from build123d import *

# Parameters (mm, degrees)
SKETCH1_R           = 4
SKETCH1_R_2         = 1
BOSS_EXTRUDE1_DEPTH = 1
FILLET1_R           = 2


with BuildPart() as part:
    # Sketch1 → Boss-Extrude1 (new body)
    with BuildSketch(Plane.XY):
        Polygon((-31.163774815, -36.354373739), (-22.29015667, -20.984816263), (-9.5, -16.574119451), (-9.5, 20), (9.5, 20), (9.5, -18.535898385), (1.11843014, -33.05320323), (12.977241336, -39.899891067), (3.477241336, -56.354373739), align=None)
        with Locations((0, 10.5)):
            Circle(SKETCH1_R, mode=Mode.SUBTRACT)
        with Locations((0, -43.377132403)):
            Circle(SKETCH1_R, mode=Mode.SUBTRACT)
        with Locations((2.745190528, -53.622322931)):
            Circle(SKETCH1_R_2, mode=Mode.SUBTRACT)
        with Locations((-28.431724008, -35.622322931)):
            Circle(SKETCH1_R_2, mode=Mode.SUBTRACT)
        with Locations((10.245190528, -40.631941874)):
            Circle(SKETCH1_R_2, mode=Mode.SUBTRACT)
        with Locations((-20.931724008, -22.631941874)):
            Circle(SKETCH1_R_2, mode=Mode.SUBTRACT)
        with Locations((-7.5, -18)):
            Circle(SKETCH1_R_2, mode=Mode.SUBTRACT)
        with Locations((7.5, -18)):
            Circle(SKETCH1_R_2, mode=Mode.SUBTRACT)
        with Locations((7.5, 18)):
            Circle(SKETCH1_R_2, mode=Mode.SUBTRACT)
        with Locations((-7.5, 18)):
            Circle(SKETCH1_R_2, mode=Mode.SUBTRACT)
    extrude(amount=BOSS_EXTRUDE1_DEPTH)

    # Fillet1
    fillet1_edges = [part.edges().sort_by_distance(p)[0] for p in [
        (-22.29015667, -20.984816263, 0.5),
        (-9.5, -16.574119451, 0.5),
        (-9.5, 20, 0.5),
        (9.5, 20, 0.5),
        (9.5, -18.535898385, 0.5),
        (1.11843014, -33.05320323, 0.5),
        (12.977241336, -39.899891067, 0.5),
        (3.477241336, -56.354373739, 0.5),
        (-31.163774815, -36.354373739, 0.5),
    ]]
    fillet(fillet1_edges, radius=FILLET1_R)


solid = part.part
Geometry check sheet. Reference: the model listing, model coordinates, mm. A direction names the side the tool comes from. Give positions to 0.01 mm unless a question says otherwise; leave off trailing zeros. Loops run counter-clockwise (first coordinate to the right, second up) from the corner with the lowest first, then second, coordinate; pieces in that order, holes last. Notation, with made-up numbers: M -24.75,28.5 L -15.75,28.5 A15 ccw -15.75,56.5 Z; hole C -38.75,-11.5 d9. An arc over 180 degrees is marked long. Answer as a JSON object with one key per item and string values. Group by question number.
Item 1: Mould release check, pull along Y, two halves, no side actions. Record for faces 3 (the cylindrical face through (8.9, 19.43, 0.51)), 4 (the cylindrical face through (2.53, -54.6, 0.49)), 5 (the flat face through (8.3, -48, 0.5)), 6 (the cylindrical face through (9.246, -40.588, 0.493)): pulls with the +Y half, pulls with the -Y half, needs draft (parallel to the pull), parting line crosses it, or undercut.
Item 2: Material ranges on L1, parallel to Y at x = 0, z = 0.3; L2, parallel to Y at x = 7.5, z = 0.75; L3, parallel to Y at x = -1, z = 0.75, recorded low to high.
Item 3: Sectioned sample at D-D on x = -18. Record the boundary of the cut face in (y, z).
Item 4: Sectioned sample at A-A on y = 11.5. Record the boundary of the cut face in (x, z), plus the area to 3 significant figures.
Item 5: Access from +Z, -Z, +X, -X, +Y, -Y to the whole of each face (thin tool, end or side, straight path). Record for faces 1 (the cylindrical face through (-7.717, -18.976, 0.493)), 2 (the flat face through (6.989, -36.443, 0.493)).
Item 6: Sectioned sample at C-C on z = 0.75. Give the number of separate pieces and of enclosed holes in the cut face, plus the area to 3 significant figures.
Item 7: Sectioned sample at B-B on x = 0. Record the boundary of the cut face in (y, z).
Findings below:
{
 "1": {"face 3": "pulls with the +Y half", "face 4": "undercut", "face 5": "pulls with the -Y half", "face 6": "undercut"},
 "2": {"L1": "-54.35 to -47.38, -39.38 to 6.5, 14.5 to 20", "L2": "-49.39 to -36.74, -22 to -19, -17 to 17, 19 to 20", "L3": "-53.77 to -47.25, -39.5 to 6.63, 14.37 to 20"},
 "3": {"outline": "M -43.95,0 L -19.51,0 L -19.51,1 L -43.95,1 Z"},
 "4": {"outline": "M -9.5,0 L -3.87,0 L -3.87,1 L -9.5,1 Z; M 3.87,0 L 9.5,0 L 9.5,1 L 3.87,1 Z", "area": "11.3 mm2"},
 "5": {"face 1": "+Z, -Z", "face 2": "+Z, -Z, +X"},
 "6": {"separate pieces": "1", "enclosed holes": "10", "area": "1,600 mm2"},
 "7": {"outline": "M -54.35,0 L -47.38,0 L -47.38,1 L -54.35,1 Z; M -39.38,0 L 6.5,0 L 6.5,1 L -39.38,1 Z; M 14.5,0 L 20,0 L 20,1 L 14.5,1 Z"}
}
